Read the model definition and answer for the solid it produces. Units are mm, in the model's axes. A direction names the side the tool comes from. Coordinates: 2 decimals unless noted, no trailing zeros. Loops run counter-clockwise (first coordinate to the right, second up) from the corner with the lowest first, then second, coordinate; pieces in that order, holes last. Notation, with made-up numbers: (-4.5, 9) -> (36.5, 9) arc R12 cw to (36.5, 23) -> close; hole circle Ø1 at (-19, 57.25). An arc over 180 degrees is marked (long way). Answer as CSV lines item,"result".
Autodesk Fusion 360 part; units mm, degrees
sketch "Sketch1" plane through (0, 0, 0) normal (0, 0, 1) x (1, 0, 0)
  line L0 (10, 52.3205) -> (0, 35)
  line L1 (0, 35) -> (0, 0)
  line L2 (0, 0) -> (5.4848, -9.5)
  line L3 (17.6092, -9.5) -> (23.094, 0)
  line L4 (14.3301, 49.8205) -> (5, 33.6603)
  line L5 (5, 33.6603) -> (5, 1.3397)
  line L6 (5, 1.3397) -> (7.2169, -2.5)
  line L7 (15.8771, -2.5) -> (18.7639, 2.5)
  line L8 (23.094, 0) -> (18.7639, 2.5)
  line L9 (14.3301, 49.8205) -> (10, 52.3205)
  arc A0 (7.2169, -2.5) -> (15.8771, -2.5) centre (11.547, 0) ccw
  arc A1 (5.4848, -9.5) -> (17.6092, -9.5) centre (11.547, -6) ccw
  point P0 (11.547, -20)
  dimension "d1" = 35
  dimension "d2" = 20
  dimension "d3" = 20
  dimension "d4" = 20
  dimension "d5" = 150
  dimension "d6" = 150
  dimension "d8" = 5
  dimension "d9" = 7
extrude "Extrude1" add sketch "Sketch1" along normal blind 15
sketch "Sketch2" plane through (5, 0, 0) normal (1, 0, 0) x (0, 0, -1)
  line L0 (0, 1.3397) -> (0, 33.6603)
  line L1 (0, 33.6603) -> (-15, 33.6603)
  line L2 (-15, 33.6603) -> (-15, 1.3397)
  line L3 (-15, 1.3397) -> (0, 1.3397)
  line L4 (-7.5, 1.3397) -> (-7.5, 33.6603) construction
  line L5 (-15, 17.5) -> (0, 17.5) construction
  circle A0 centre (-7.5, 26.7565) radius 4
  circle A1 centre (-7.5, 8.2435) radius 4
  dimension "d12" = 8
  dimension "d13" = 6.9037
extrude "Extrude2" cut sketch "Sketch2" against normal blind 3 draft -35 contours A0 | A1
extrude "Extrude3" cut 2 faces at (2, 27.3459, 7.7313) (2, 8.7385, 7.1999) along direction (-1, 0, 0) through all
fillet "Fillet1" radius 7.5 4 edges at (20.9289, 1.25, 15) (20.9289, 1.25, 0) (12.1651, 51.0705, 15) (12.1651, 51.0705, 0)
fillet "Fillet2" radius 8 4 edges at (5, 1.3397, 7.5) (0, 0, 7.5) (0, 35, 7.5) (5, 33.6603, 7.5)
fillet "Fillet3" radius 0.5 16 edges at (5.2726, 33.5872, 15) (8.326, 39.421, 15) (14.3301, 49.8205, 7.5) (8.326, 39.421, 0) (5.2726, 33.5872, 0) (5, 17.5, 0) (5.2726, 1.4128, 0) (6.6443, -1.5083, 0) (10.6702, -4.9225, 0) (15.3815, -3.2072, 0.0512) (18.7639, 2.5, 7.5) (15.3815, -3.2072, 14.9488) (10.6702, -4.9225, 15) (6.6443, -1.5083, 15) (5.2726, 1.4128, 15) (5, 17.5, 15)
equation "d3 = d2"
equation "d4 = d2"
equation "d6 = d5"
Q1. For faces 5 (the face through (6.636, -1.494, 7.402)), 6 (the face through (19.87, -0.74, 12.86)), 7 (the face through (10.132, 42.549, 7.402)), determine the directions among +Z, -Z, +X, -X, +Y, -Y from which every point of the face is accessible in a straight line to the end or side of a thin tool.
Results:
face 5,"+Z, -Z"
face 6,"+Z, +X, +Y"
face 7,"+Z, -Z, +X"
Q2. Find the intervals of material crossed by probe 1 along X at (y, z) = (13, 1.5); probe 2 along Y at (x, z) = (11.75, 3.5); probe 3 along X at (y, z) = (25, 10.5), in increasing order. Write a range as [from, to].
Results:
probe 1,"x = [0, 5]"
probe 2,"y = [-13, -5], [45.35, 49.98]"
probe 3,"x = [0, 4.25]"
Q3. Given pin 1 Ø5 at (y, z) = (41, 6) entering from -X; pin 2 Ø4 at (x, z) = (10.5, 5) entering from +Y; pin 3 Ø7 at (y, z) = (24.5, 8) entering from +X, each flat-ended and moving along its own axis, determine where each tip first touches the part or whether it passes through.
Results:
pin 1,"stops at x = 2.02"
pin 2,"stops at y = 52.3"
pin 3,"stops at x = 5"
Q4. A cutting plane is placed at B-B, the plane x = 3.75. Write down the section's boundary in (y, z).
Results:
outline,"(-6.5, 0) -> (41.5, 0) -> (41.5, 15) -> (-6.5, 15) -> close; hole circle Ø6.25 at (8.24, 7.5); hole circle Ø6.25 at (26.76, 7.5)"
Q5. A cutting plane is placed at A-A, the plane y = 17. Write down the section's boundary in (x, z), and give its area (3 significant figures).
Results:
outline,"(0, 0) -> (4.5, 0) arc R0.5 ccw to (5, 0.5) -> (5, 14.5) arc R0.5 ccw to (4.5, 15) -> (0, 15) -> close"
area,"74.9 mm²"
Q6. For a pull along Z with two mould halves and no side action, classify faces 1 (the face through (8.234, 39.548, 0.15)), 2 (the face through (4, 12, 15)), 3 (the face through (1.014, 7.516, 5.745)), 4 (the face through (0.28, 34.96, 7.6)) as pulls with the +Z half, pulls with the -Z half, needs draft (parallel to the pull), parting line crosses it, or undercut.
Results:
face 1,"pulls with the -Z half"
face 2,"pulls with the +Z half"
face 3,"undercut"
face 4,"needs draft"
